Source: CAD feature listing. Evaluate the final solid. Frame: model axes, mm. A direction names the side the tool comes from. Give positions to 0.01 mm unless a question says otherwise; leave off trailing zeros. Loops run counter-clockwise (first coordinate to the right, second up) from the corner with the lowest first, then second, coordinate; pieces in that order, holes last.
Solid Edge part; units mm, degrees
sketch "Sketch1" plane through (0, 0, 0) normal (0, 0, 1) x (1, 0, 0)
  line L0 (35.8429, 70) -> (36.8928, 82)
  line L1 (33.7303, 82) -> (36.8928, 82)
  line L2 (19.6963, 2.409) -> (33.7303, 82)
  line L3 (0, 2.409) -> (19.6963, 2.409)
  line L4 (0, 0) -> (0, 2.409)
  line L5 (0, 0) -> (21.5, 0)
  line L6 (21.5, 0) -> (33.8429, 70)
  line L7 (33.8429, 70) -> (35.8429, 70)
revolve "RevolvedProtrusion1" add sketch "Sketch1" angle 360 about axis through (0, 82, 0) along (0, -1, 0)
properties material "Polietileno, baja densidad"
(1) Ray query, line 1 along X through (y, z) = (66, -17); line 2 along X through (y, z) = (40.5, -4); line 3 along Z through (x, y) = (-20.5, 31.5). Return the intervals inside material, ascending.
A:
line 1: x = -28.44 to -25.81, 25.81 to 28.44
line 2: x = -28.36 to -26.11, 26.11 to 28.36
line 3: z = -17.65 to -14, 14 to 17.65
(2) Section C-C, the plane y = 14. Return the cut outline in (x, z).
A:
outline: circle Ø47.94 at (0, 0); hole circle Ø43.48 at (0, 0)
(3) Reachability of faces 5 (the flat face through (32, 70, -13)), 6 (the flat face through (0, 0, 0)) from +Z, -Z, +X, -X, +Y, -Y: full face, straight path, thin tool, end or side. Return the list, or none.
A:
face 5: -Y
face 6: +Z, -Z, +X, -X, -Y
(4) Mould query, pull axis Z, two halves, no side actions, for faces 1 (the flat face through (0, 2.409, 0)), 2 (the flat face through (16, 82, -30)), 3 (the conical face through (-5.474, 33.918, 24.652)), 4 (the conical face through (34.47, 73.42, -10.86)). Classes: pulls with the +Z half, pulls with the -Z half, needs draft (parallel to the pull), parting line crosses it, or undercut.
A:
face 1: undercut
face 2: needs draft
face 3: undercut
face 4: parting line crosses it
(5) First-contact query: pin 1 (2 mm diameter, centred on y = 65.5, z = 4, fed in from -X); pin 2 (6 mm diameter, centred on y = 59, z = -20, fed in from -X); pin 3 (8 mm diameter, centred on y = 58, z = 24, fed in from +X). Flat tips, straight axial feed; report the tip coordinate or a pass-through.
A:
pin 1: stops at x = -33.02
pin 2: stops at x = -27.1
pin 3: stops at x = 24.75
(6) Section B-B, the plane z = 0. Return the cut outline in (x, y).
A:
outline: (-36.89, 82) - (-35.84, 70) - (-33.84, 70) - (-21.5, 0) - (21.5, 0) - (33.84, 70) - (35.84, 70) - (36.89, 82) - (33.73, 82) - (19.7, 2.41) - (-19.7, 2.41) - (-33.73, 82) - close
(7) Section A-A, the plane x = 0. Return the cut outline in (y, z).
A:
outline: (0, -21.5) - (70, -33.84) - (70, -35.84) - (82, -36.89) - (82, -33.73) - (2.41, -19.7) - (2.41, 19.7) - (82, 33.73) - (82, 36.89) - (70, 35.84) - (70, 33.84) - (0, 21.5) - close
(8) Section D-D, the plane y = 45.5. Return the cut outline in (x, z).
A:
outline: circle Ø59.05 at (0, 0); hole circle Ø54.59 at (0, 0)
